from build123d import *

# Parameters (mm, degrees)
SKETCH1_R           = 155
BOSS_EXTRUDE1_DEPTH = 1
SKETCH2_W           = 9.944482202
SKETCH2_H           = 9.944482203
BOSS_EXTRUDE2_DEPTH = 0.1


with BuildPart() as part:
    # Sketch1 → Boss-Extrude1 (new body)
    with BuildSketch(Plane.XY):
        Circle(SKETCH1_R)
    extrude(amount=BOSS_EXTRUDE1_DEPTH)

    # Sketch2 → Boss-Extrude2 (add)
    with BuildSketch(Plane.XY.offset(1)):
        with Locations((-10, 13.832433297)):
            Rectangle(SKETCH2_W, SKETCH2_H)
        with Locations((6, 13.832433297)):
            Rectangle(SKETCH2_W, SKETCH2_H)
        with BuildLine():
            Line((-13.779336212, 2.051462451), (-13.779336212, 0))
            ThreePointArc((-13.779336212, 0), (-14.972241101, -1.19290489), (-16.165145991, 0))
            Line((-16.165145991, 0), (-16.165145991, 2.051462451))
            ThreePointArc((-16.165145991, 2.051462451), (-14.972241101, 3.244367341), (-13.779336212, 2.051462451))
        make_face()
        with BuildLine():
            Line((-16.165145991, -6.802865473), (-16.165145991, -4.751403022))
            ThreePointArc((-16.165145991, -4.751403022), (-14.972241101, -3.558498133), (-13.779336212, -4.751403022))
            Line((-13.779336212, -4.751403022), (-13.779336212, -6.802865473))
            ThreePointArc((-13.779336212, -6.802865473), (-14.972241101, -7.995770363), (-16.165145991, -6.802865473))
        make_face()
        with BuildLine():
            Line((-0.185839603, -15.881052977), (-0.185839603, -17.932515427))
            ThreePointArc((-0.185839603, -17.932515427), (-1.378744492, -19.125420317), (-2.571649382, -17.932515427))
            Line((-2.571649382, -17.932515427), (-2.571649382, -15.881052977))
            ThreePointArc((-2.571649382, -15.881052977), (-1.378744492, -14.688148087), (-0.185839603, -15.881052977))
        make_face()
        with BuildLine():
            Line((3.900067015, -15.881052977), (3.900067015, -17.932515427))
            ThreePointArc((3.900067015, -17.932515427), (2.707162125, -19.125420317), (1.514257236, -17.932515427))
            Line((1.514257236, -17.932515427), (1.514257236, -15.881052977))
            ThreePointArc((1.514257236, -15.881052977), (2.707162125, -14.688148087), (3.900067015, -15.881052977))
        make_face()
        with BuildLine():
            Line((-0.185839603, -21.393622173), (-0.185839603, -23.445084624))
            ThreePointArc((-0.185839603, -23.445084624), (-1.378744492, -24.637989514), (-2.571649382, -23.445084624))
            Line((-2.571649382, -23.445084624), (-2.571649382, -21.393622173))
            ThreePointArc((-2.571649382, -21.393622173), (-1.378744492, -20.200717283), (-0.185839603, -21.393622173))
        make_face()
        with BuildLine():
            Line((1.514257236, -23.445084624), (1.514257236, -21.393622173))
            ThreePointArc((1.514257236, -21.393622173), (2.707162125, -20.200717283), (3.900067015, -21.393622173))
            Line((3.900067015, -21.393622173), (3.900067015, -23.445084624))
            ThreePointArc((3.900067015, -23.445084624), (2.707162125, -24.637989514), (1.514257236, -23.445084624))
        make_face()
    extrude(amount=BOSS_EXTRUDE2_DEPTH)


solid = part.part
Could you check a few things on this model? Use its own coordinates, in mm. Give positions to 0.01 mm unless a question says otherwise; leave off trailing zeros. Order: outer loops, then holes, each group sorted by start corner. A loop starts at its lowest first (then second) coordinate and runs counter-clockwise, first axis right, second up. Notation, with made-up numbers: M 11.5,-28 L 19.5,-28 A13 cw 19.5,-10 Z; hole C 27,76.25 d2. An arc over 180 degrees is marked long. One line per question, with ' | ' between items.
1. If I drill on line 1 (Z direction, x = -80, y = -106); line 2 (X direction, y = 134.5, z = 0.7); line 3 (X direction, y = -100, z = 0.8), over which ranges is the centre line in solid material (lowest first)?
Results:
line 1: 0 to 1 | line 2: -77.04 to 77.04 | line 3: -118.43 to 118.43
2. I want a section at C-C (y = -34.5). List the corners of the cut face in (x, z) for me, and give its area (3 significant figures).
Results:
outline: M -151.11,0 L 151.11,0 L 151.11,1 L -151.11,1 Z | area: 302 mm²
3. I want a section at B-B (x = -27.5). List the corners of the cut face in (y, z) for me, and give its area (3 significant figures).
Results:
outline: M -152.54,0 L 152.54,0 L 152.54,1 L -152.54,1 Z | area: 305 mm²
4. I want a section at A-A (z = 0.45). List the corners of the cut face in (x, y) for me, and give its area (3 significant figures).
Results:
outline: C 0,0 d310 | area: 75,500 mm²
5. I'm going to push flat-ended pins straight in: pin 1 (3 mm diameter, centred on x = -118, y = -69.5, fed in from +Z); pin 2 (5 mm diameter, centred on x = 50.5, y = 43.5, fed in from -Z). Where does each tip first touch, or does it pass through?
Results:
pin 1: z = 1 | pin 2: z = 0
